Could you check a few things on this model? Use its own coordinates, in mm. Face numbers are marked on the shaded views. Give positions to 0.01 mm unless a question says otherwise; leave off trailing zeros. Order: outer loops, then holes, each group sorted by start corner. A loop starts at its lowest first (then second) coordinate and runs counter-clockwise, first axis right, second up.
from build123d import *

# Parameters (mm, degrees)
F2_DEPTH = 12.7
F3_DEPTH = 25.4


with BuildPart() as f2:
    # F1 (on Front) → F2 (new body)
    with BuildSketch(Plane.XZ):
        with BuildLine():
            Line((150.01875, 28.475608), (-1.322917, 15.819782))
            ThreePointArc((-1.322917, 15.819782), (-15.874999, 0), (-1.322917, -15.819782))
            Line((-1.322917, -15.819782), (150.01875, -28.475608))
            ThreePointArc((150.01875, -28.475608), (180.974999, 0), (150.01875, 28.475608))
        make_face()
    extrude(amount=F2_DEPTH)

    # F0 (on Front) → F3 (cut)
    with BuildSketch(Plane.XZ):
        with BuildLine():
            Line((150.547917, 22.147695), (-0.79375, 9.491869))
            ThreePointArc((-0.79375, 9.491869), (-9.525, 0), (-0.79375, -9.491869))
            Line((-0.79375, -9.491869), (150.547917, -22.147695))
            ThreePointArc((150.547917, -22.147695), (174.625, 0), (150.547917, 22.147695))
        make_face()
    extrude(amount=F3_DEPTH, mode=Mode.SUBTRACT)


solid = f2.part
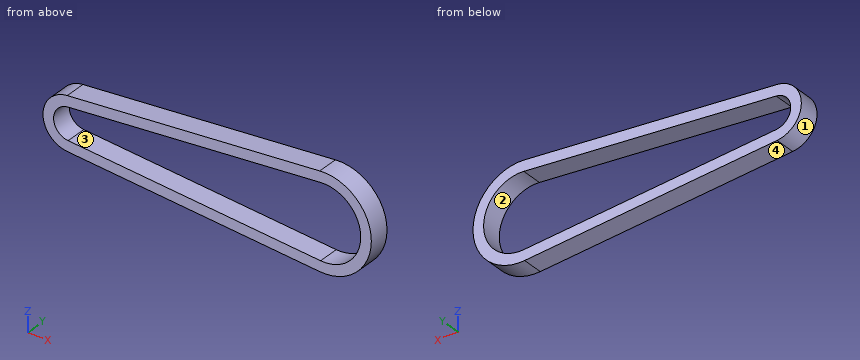
Item 1: Imagine slicing it at C-C on y = -5.75. List the corners of the cut face in (x, z) for me (3 decimals), then the cut area to 3 significant figures.
Findings:
outline: (-1.323, -15.82) - (150.019, -28.476) arc R28.575 ccw (long way) to (150.019, 28.476) - (-1.323, 15.82) arc R15.875 ccw to start; hole (-0.794, -9.492) - (150.548, -22.148) arc R22.225 ccw (long way) to (150.548, 22.148) - (-0.794, 9.492) arc R9.525 ccw to start
area: 2,700 mm2
Item 2: Imagine slicing it at B-B on z = 0. List the corners of the cut face in (x, y) for me (3 decimals), then the cut area to 3 significant figures.
Findings:
outline: (-15.875, -12.7) - (-9.525, -12.7) - (-9.525, 0) - (-15.875, 0) - close; (174.625, -12.7) - (180.975, -12.7) - (180.975, 0) - (174.625, 0) - close
area: 161 mm2
Item 3: Please list where these lines run through material, in increasing order: line 1 along Z through (x, y) = (152.4, -3.25) (3 decimals); line 2 along Z through (x, y) = (72.5, -6.25); line 3 along X through (y, z) = (-5.5, 7).
Findings:
line 1: z = -28.575 to -22.225, 22.225 to 28.575
line 2: z = -21.99 to -15.62, 15.62 to 21.99
line 3: x = -14.25 to -6.46, 173.49 to 180.1
Item 4: For pin 1 (6 mm diameter, centred on y = -9, z = -12, fed in from -X); pin 2 (1.5 mm diameter, centred on y = -4.5, z = 0.5, fed in from -X) (3 decimals); pin 3 (3 mm diameter, centred on y = -5.5, z = -8.5, fed in from +X); pin 4 (1 mm diameter, centred on y = -4.5, z = -15, fed in from -X), each with a flat end and sliding along its axis, tell me the tip position at first contact or that it passes through.
Findings:
pin 1: stops at x = -13.08
pin 2: stops at x = -15.875
pin 3: stops at x = 180.1
pin 4: stops at x = -6.46
Item 5: We'd pull the mould along Z, two halves only. Please class the marked faces 1, 2, 3 and 4: +Z half, -Z half, draft (parallel to the pull), parting line (faces both ways), or undercut.
Findings:
face 1: parting line
face 2: undercut
face 3: undercut
face 4: -Z half
Item 6: Imagine slicing it at A-A on x = 152.4. List the corners of the cut face in (y, z) for me (3 decimals).
Findings:
outline: (-12.7, -28.575) - (0, -28.575) - (0, -22.225) - (-12.7, -22.225) - close; (-12.7, 22.225) - (0, 22.225) - (0, 28.575) - (-12.7, 28.575) - close
